For this review, take the finished solid that the model builds, in its own axes (mm). A direction names the side the tool comes from. Give positions to 0.01 mm unless a question says otherwise; leave off trailing zeros. Loops run counter-clockwise (first coordinate to the right, second up) from the corner with the lowest first, then second, coordinate; pieces in that order, holes last. Notation, with made-up numbers: (23, 73) - (68, 73) arc R31 ccw to (68, 108) - close; hole circle Ø6 at (9, 40.25). An arc over 180 degrees is marked (long way). Use CSV: the item, a comma, the result in double quotes. Start each with the question number.
1. Take a section at C-C on y = 2.5. Give the boundary of the cut face in (x, z), plus the area to 3 significant figures.
2. Take a section at B-B on x = 0. Give the boundary of the cut face in (y, z), plus the area to 3 significant figures.
3. Take a section at D-D on x = -11.5. State how many separate pieces and enclosed holes the cut face has, plus the area to 3 significant figures.
4. For faces 1 (the cylindrical face through (-11.99, 25.49, -0.53)), 2 (the cylindrical face through (-2.539, 4.93, -19.334)), 3 (the flat face through (5.2, 20, -0.2)), list the 3-axis set-ups (+Z, -Z, +X, -X, +Y, -Y) from which the entire face can be reached by the end or side of a thin tool; tool diameter is ignored.
5. Wall thickness on line 1 (Y direction, x = -2.5, z = 9.5); line 2 (Y direction, x = -13, z = 4); line 3 (Y direction, x = 9, z = -17): over which ranges is each line inside the solid? List them lowest first.
6. For pin 1 (3 mm diameter, centred on x = -2, y = 5.5, fed in from -Z); pin 2 (12 mm diameter, centred on x = 1.5, y = 12, fed in from +Z); pin 3 (1.5 mm diameter, centred on x = 5, y = 11, fed in from +Z), all flat-tipped, find the tip position at first contact; note any pin that passes through.
7. Mouldability with a two-part tool opening along Y and no side actions: class faces 4 (the flat face through (18.7, 10, 4.2)), 5 (the flat face through (4, 15, 4)), 6 (the cylindrical face through (-11.99, 20.49, -0.53)) as pulls with the +Y half, pulls with the -Y half, needs draft (parallel to the pull), parting line crosses it, or undercut.
8. Take a section at A-A on z = 0. Give the boundary of the cut face in (x, y).
```python
from build123d import *

# Parameters (mm, degrees)
SKETCH_1_R      = 19.5
EXTRUDE_1_DEPTH = 10
SKETCH_2_R      = 19
EXTRUDE_2_DEPTH = 5
SKETCH_3_R      = 5
EXTRUDE_3_DEPTH = 5


with BuildPart() as part:
    # 草图1 → 凸台-拉伸1 (new body)
    with BuildSketch(Plane(origin=(0, 0, 0), x_dir=(1, 0, 0), z_dir=(0, 1, 0))):
        Circle(SKETCH_1_R)
    extrude(amount=EXTRUDE_1_DEPTH)

    # 草图2 → 凸台-拉伸2 (add)
    with BuildSketch(Plane(origin=(0, 10, 0), x_dir=(1, 0, 0), z_dir=(0, 1, 0))):
        Circle(SKETCH_2_R)
    extrude(amount=EXTRUDE_2_DEPTH)

    # 草图3 → 凸台-拉伸3 (add)
    with BuildSketch(Plane(origin=(0, 15, 0), x_dir=(1, 0, 0), z_dir=(0, 1, 0))):
        Circle(SKETCH_3_R)
    extrude(amount=EXTRUDE_3_DEPTH)

    # 草图5 → 旋转1 (revolve)
    with BuildSketch(Plane.XY):
        with BuildLine():
            Line((0, 20), (0, 26))
            Line((0, 26), (12, 26))
            Line((12, 26), (12, 25))
            ThreePointArc((12, 25), (11, 23), (12, 21))
            Line((12, 21), (12, 20))
            Line((12, 20), (0, 20))
        make_face()
    revolve(axis=Axis((0, 20, 0), (0, 1, 0)))


solid = part.part
```
Check result:
1,outline,"circle Ø39 at (0, 0)"
1,area,"1,190 mm²"
2,outline,"(0, -19.5) - (10, -19.5) - (10, -19) - (15, -19) - (15, -5) - (20, -5) - (20, -12) - (21, -12) arc R2.5 cw to (25, -12) - (26, -12) - (26, 12) - (25, 12) arc R2.5 cw to (21, 12) - (20, 12) - (20, 5) - (15, 5) - (15, 19) - (10, 19) - (10, 19.5) - (0, 19.5) - close"
2,area,"768 mm²"
3,separate pieces,"3"
3,enclosed holes,"0"
3,area,"484 mm²"
4,face 1,"+Y"
4,face 2,"+Y, -Y"
4,face 3,"none"
5,line 1,"y = 0 to 15, 20 to 26"
5,line 2,"y = 0 to 15"
5,line 3,"y = 0 to 10"
6,pin 1,"stops at z = -19.49"
6,pin 2,"stops at z = 19.5"
6,pin 3,"stops at z = 18.52"
7,face 4,"pulls with the +Y half"
7,face 5,"undercut"
7,face 6,"needs draft"
8,outline,"(-19.5, 0) - (19.5, 0) - (19.5, 10) - (19, 10) - (19, 15) - (5, 15) - (5, 20) - (12, 20) - (12, 21) arc R2.5 cw to (12, 25) - (12, 26) - (-12, 26) - (-12, 25) arc R2.5 cw to (-12, 21) - (-12, 20) - (-5, 20) - (-5, 15) - (-19, 15) - (-19, 10) - (-19.5, 10) - close"
